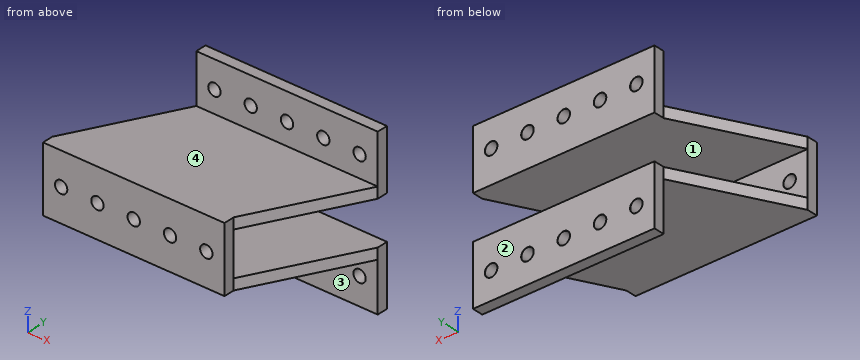
```python
from build123d import *

# Parameters (mm, degrees)
SKETCH1_W                      = 49.9999
SKETCH1_H                      = 14.9999999
BOSS_EXTRUDE1_DEPTH            = 3
BOSS_EXTRUDE2_START            = 35
SKETCH1_3_W                    = 49.9999
SKETCH1_3_H                    = 14.9999999
BOSS_EXTRUDE2_DEPTH            = 3
BOSS_EXTRUDE2_2_DEPTH          = 3
M3_CLEARANCE_HOLE1_AT_2_COUNT  = 2
M3_CLEARANCE_HOLE1_AT_2_PITCH  = 36.055512588
M3_CLEARANCE_HOLE1_AT_3_COUNT  = 2
M3_CLEARANCE_HOLE1_AT_3_PITCH  = 20
M3_CLEARANCE_HOLE1_AT_4_COUNT  = 2
M3_CLEARANCE_HOLE1_AT_4_PITCH  = 42.42640673
M3_CLEARANCE_HOLE1_AT_5_COUNT  = 2
M3_CLEARANCE_HOLE1_AT_5_PITCH  = 30
M3_CLEARANCE_HOLE1_AT_6_COUNT  = 2
M3_CLEARANCE_HOLE1_AT_6_PITCH  = 49.99999988
M3_CLEARANCE_HOLE1_AT_7_COUNT  = 2
M3_CLEARANCE_HOLE1_AT_7_PITCH  = 40
M3_CLEARANCE_HOLE1_AT_8_COUNT  = 2
M3_CLEARANCE_HOLE1_AT_8_PITCH  = 31.622776412
M3_CLEARANCE_HOLE1_AT_9_COUNT  = 2
M3_CLEARANCE_HOLE1_AT_9_PITCH  = 10
M3_CLEARANCE_HOLE1_AT_10_COUNT = 2
M3_CLEARANCE_HOLE1_AT_10_PITCH = 29.9999998
M3_CLEARANCE_HOLE2_AT_2_COUNT  = 2
M3_CLEARANCE_HOLE2_AT_2_PITCH  = 20
M3_CLEARANCE_HOLE2_AT_3_COUNT  = 2
M3_CLEARANCE_HOLE2_AT_3_PITCH  = 30
M3_CLEARANCE_HOLE2_AT_4_COUNT  = 2
M3_CLEARANCE_HOLE2_AT_4_PITCH  = 40
M3_CLEARANCE_HOLE2_AT_5_COUNT  = 2
M3_CLEARANCE_HOLE2_AT_5_PITCH  = 10
BOSS_EXTRUDE3_DEPTH            = 1.5
BOSS_EXTRUDE3_DEPTH_BACK       = 1.5
BOSS_EXTRUDE4_DEPTH            = 1.5
BOSS_EXTRUDE4_DEPTH_BACK       = 1.5
BOSS_EXTRUDE4_START            = -15


with BuildPart() as part:
    # Sketch1 → Boss-Extrude1 (new body)
    with BuildSketch(Plane(origin=(0, 0, 0), x_dir=(1, 0, 0), z_dir=(0, 1, 0))):
        with Locations((24.99995, 22.49999985)):
            Rectangle(SKETCH1_W, SKETCH1_H)
    extrude(amount=BOSS_EXTRUDE1_DEPTH)

    # Sketch8 → M3 Clearance Hole2 (revolve, cut)
    with BuildSketch(Plane(origin=(4.99995, 3, -22.49999985), x_dir=(0, 0, 1), z_dir=(1, 0, 0))):
        Polygon((0, 0), (0, 3), (1.7, 3), (1.7, 0.025), (1.725, 0), align=None)
    m3_clearance_hole2 = revolve(axis=Axis((4.99995, 9.35, -22.49999985), (0, -1, 0)), mode=Mode.SUBTRACT)

    # M3 Clearance Hole2 at 2: M3 Clearance Hole2 ×2
    with Locations(*[(i * M3_CLEARANCE_HOLE2_AT_2_PITCH, 0, 0) for i in range(1, M3_CLEARANCE_HOLE2_AT_2_COUNT)]):
        add(m3_clearance_hole2, mode=Mode.SUBTRACT)

    # M3 Clearance Hole2 at 3: M3 Clearance Hole2 ×2
    with Locations(*[(i * M3_CLEARANCE_HOLE2_AT_3_PITCH, 0, 0) for i in range(1, M3_CLEARANCE_HOLE2_AT_3_COUNT)]):
        add(m3_clearance_hole2, mode=Mode.SUBTRACT)

    # M3 Clearance Hole2 at 4: M3 Clearance Hole2 ×2
    with Locations(*[(i * M3_CLEARANCE_HOLE2_AT_4_PITCH, 0, 0) for i in range(1, M3_CLEARANCE_HOLE2_AT_4_COUNT)]):
        add(m3_clearance_hole2, mode=Mode.SUBTRACT)

    # M3 Clearance Hole2 at 5: M3 Clearance Hole2 ×2
    with Locations(*[(i * M3_CLEARANCE_HOLE2_AT_5_PITCH, 0, 0) for i in range(1, M3_CLEARANCE_HOLE2_AT_5_COUNT)]):
        add(m3_clearance_hole2, mode=Mode.SUBTRACT)



with BuildPart() as body_2:
    # Sketch1<3> → Boss-Extrude2 (new body)
    with BuildSketch(Plane(origin=(0, 0, 0), x_dir=(1, 0, 0), z_dir=(0, 1, 0)).offset(BOSS_EXTRUDE2_START)):
        with Locations((39.99895, 37.49999975)):
            Rectangle(SKETCH1_3_W, SKETCH1_3_H)
    extrude(amount=-BOSS_EXTRUDE2_DEPTH)


with BuildPart() as body_3:
    # Sketch1<3> → Boss-Extrude2 2 (new body)
    with BuildSketch(Plane(origin=(0, 0, 0), x_dir=(1, 0, 0), z_dir=(0, 1, 0)).offset(BOSS_EXTRUDE2_START)):
        with Locations((39.99895, 7.49999995)):
            Rectangle(SKETCH1_3_W, SKETCH1_3_H)
    extrude(amount=-BOSS_EXTRUDE2_2_DEPTH)

    # Sketch6 → M3 Clearance Hole1 (revolve, cut)
    with BuildSketch(Plane(origin=(19.99895, 35, -7.49999995), x_dir=(0, 0, 1), z_dir=(1, 0, 0))):
        Polygon((0, 0), (0, 35), (1.7, 35), (1.7, 0.025), (1.725, 0), align=None)
    m3_clearance_hole1 = revolve(axis=Axis((19.99895, 41.35, -7.49999995), (0, -1, 0)), mode=Mode.SUBTRACT)

    # M3 Clearance Hole1 at 3: M3 Clearance Hole1 ×2
    with Locations(*[(i * M3_CLEARANCE_HOLE1_AT_3_PITCH, 0, 0) for i in range(1, M3_CLEARANCE_HOLE1_AT_3_COUNT)]):
        add(m3_clearance_hole1, mode=Mode.SUBTRACT)

    # M3 Clearance Hole1 at 5: M3 Clearance Hole1 ×2
    with Locations(*[(i * M3_CLEARANCE_HOLE1_AT_5_PITCH, 0, 0) for i in range(1, M3_CLEARANCE_HOLE1_AT_5_COUNT)]):
        add(m3_clearance_hole1, mode=Mode.SUBTRACT)

    # M3 Clearance Hole1 at 7: M3 Clearance Hole1 ×2
    with Locations(*[(i * M3_CLEARANCE_HOLE1_AT_7_PITCH, 0, 0) for i in range(1, M3_CLEARANCE_HOLE1_AT_7_COUNT)]):
        add(m3_clearance_hole1, mode=Mode.SUBTRACT)

    # M3 Clearance Hole1 at 9: M3 Clearance Hole1 ×2
    with Locations(*[(i * M3_CLEARANCE_HOLE1_AT_9_PITCH, 0, 0) for i in range(1, M3_CLEARANCE_HOLE1_AT_9_COUNT)]):
        add(m3_clearance_hole1, mode=Mode.SUBTRACT)


with BuildPart() as body_2_1:
    add(body_2.part)

    # M3 Clearance Hole1 at 2: M3 Clearance Hole1 ×2
    with Locations(*[Vector(0.5547001987853687, 0, -0.832050292631084) * (i * M3_CLEARANCE_HOLE1_AT_2_PITCH) for i in range(1, M3_CLEARANCE_HOLE1_AT_2_COUNT)]):
        add(m3_clearance_hole1, mode=Mode.SUBTRACT)

    # M3 Clearance Hole1 at 4: M3 Clearance Hole1 ×2
    with Locations(*[Vector(0.7071067835435565, 0, -0.7071067788295387) * (i * M3_CLEARANCE_HOLE1_AT_4_PITCH) for i in range(1, M3_CLEARANCE_HOLE1_AT_4_COUNT)]):
        add(m3_clearance_hole1, mode=Mode.SUBTRACT)

    # M3 Clearance Hole1 at 6: M3 Clearance Hole1 ×2
    with Locations(*[Vector(0.8000000019199883, 0, -0.5999999974400156) * (i * M3_CLEARANCE_HOLE1_AT_6_PITCH) for i in range(1, M3_CLEARANCE_HOLE1_AT_6_COUNT)]):
        add(m3_clearance_hole1, mode=Mode.SUBTRACT)

    # M3 Clearance Hole1 at 8: M3 Clearance Hole1 ×2
    with Locations(*[Vector(0.3162277679141873, 0, -0.948683297418064) * (i * M3_CLEARANCE_HOLE1_AT_8_PITCH) for i in range(1, M3_CLEARANCE_HOLE1_AT_8_COUNT)]):
        add(m3_clearance_hole1, mode=Mode.SUBTRACT)

    # M3 Clearance Hole1 at 10: M3 Clearance Hole1 ×2
    with Locations(*[(0, 0, -i * M3_CLEARANCE_HOLE1_AT_10_PITCH) for i in range(1, M3_CLEARANCE_HOLE1_AT_10_COUNT)]):
        add(m3_clearance_hole1, mode=Mode.SUBTRACT)


with BuildPart() as part_1:
    add(part.part)

    add(body_3.part)  # Boss-Extrude3 merges body 3
    # Sketch2 → Boss-Extrude3 (add, two sides: drawn at the far end of the back side and taken through both)
    with BuildSketch(Plane.XY.offset(-14.9999999).offset(-BOSS_EXTRUDE3_DEPTH_BACK)):
        Polygon((0, 0), (49.9999, 0), (49.9999, 3), (64.9989, 32), (64.9989, 35), (14.999, 35), (14.999, 32), (0, 3), align=None)
    extrude(amount=BOSS_EXTRUDE3_DEPTH + BOSS_EXTRUDE3_DEPTH_BACK)


    add(body_2_1.part)  # Boss-Extrude4 merges body 2
    # Sketch2<2> → Boss-Extrude4 (add, two sides: drawn at the far end of the back side and taken through both)
    with BuildSketch(Plane.XY.offset(-14.9999999).offset(BOSS_EXTRUDE4_START - BOSS_EXTRUDE4_DEPTH_BACK)):
        Polygon((0, 0), (49.9999, 0), (49.9999, 3), (64.9989, 32), (64.9989, 35), (14.999, 35), (14.999, 32), (0, 3), align=None)
    extrude(amount=BOSS_EXTRUDE4_DEPTH + BOSS_EXTRUDE4_DEPTH_BACK)


solid = part_1.part
```
Verification items for the finished model (mm, model axes). Face numbers are marked on the shaded views. A direction names the side the tool comes from. Coordinates: 2 decimals unless noted, no trailing zeros. Write each loop counter-clockwise with the first axis right and the second up, starting at its lowest first coordinate (ties: lowest second). Pieces come first, ordered by that corner, then holes. Notation, with made-up numbers: (34.25, 72.25) - (45.25, 72.25) arc R23 ccw to (45.25, 83.25) - close; hole circle Ø6 at (47.5, -3.5). An arc over 180 degrees is marked (long way). Write item = value, one per line.
Q1. Cross-section at D-D (z = -5). Enter the section's corners in (x, y), plus the area to 3 significant figures.
Answer:
outline = (15, 32) - (65, 32) - (65, 35) - (15, 35) - close
area = 150 mm²
Q2. Cross-section at B-B (x = 53.5). Enter the section's corners in (y, z), plus the area to 3 significant figures.
Answer:
outline = (9.77, -31.5) - (32, -31.5) - (32, -45) - (35, -45) - (35, -28.5) - (9.77, -28.5) - close; (9.77, -16.5) - (35, -16.5) - (35, 0) - (32, 0) - (32, -13.5) - (9.77, -13.5) - close
area = 232 mm²
Q3. Cross-section at C-C (y = 5). Enter the section's corners in (x, z).
Answer:
outline = (1.03, -31.5) - (51.03, -31.5) - (51.03, -28.5) - (1.03, -28.5) - close; (1.03, -16.5) - (51.03, -16.5) - (51.03, -13.5) - (1.03, -13.5) - close
Q4. Material ranges on L1, parallel to Z at x = 50, y = 33; L2, parallel to X at y = 1.5, z = -22.5; L3, parallel to Z at x = 23.5, y = 32.5, recorded low to high. Write a range as from..to.
Answer:
L1 = -45..-39.2, -35.8..-28.5, -16.5..-9.2, -5.8..0
L2 = 0..3.3, 6.7..13.3, 16.7..23.3, 26.7..33.3, 36.7..43.3, 46.7..50
L3 = -45..-28.5, -16.5..0
Q5. Access from +Z, -Z, +X, -X, +Y, -Y to the whole of each face (thin tool, end or side, straight path). Record for the marked faces 1, 2, 3 and 4.
Answer:
face_1 = +X, -X, +Y
face_2 = +Z, -Z, +X, -X, +Y
face_3 = -Z, +X, -X, -Y
face_4 = +Z, +X, -X, -Y
Q6. Go/stop test with flat-tipped pins: pin 1 Ø4 at (x, z) = (44.5, -25) entering from +Y; pin 2 Ø4.5 at (x, z) = (20, -7.5) entering from -Y; pin 3 Ø6 at (x, y) = (25.5, 6) entering from +Z. Record where each tip stops, or that it passes through.
Answer:
pin_1 = 3
pin_2 = 32
pin_3 = -13.5
Q7. Cross-section at A-A (z = -22.5). Give the number of separate pieces and of enclosed holes in the cut face, plus the area to 3 significant figures.
Answer:
separate_pieces = 6
enclosed_holes = 0
area = 99.0 mm²
